from build123d import *

# Parameters (mm, degrees)
SKETCH1_R     = 4.7625
SKETCH1_R_2   = 4.0513
SHAFT_DEPTH   = 304.8
CUTAWAY_DEPTH = 305.874404981


with BuildPart() as part:
    # Sketch1 → Shaft (new body)
    with BuildSketch(Plane(origin=(0, 0, 0), x_dir=(1, 0, 0), z_dir=(0, 1, 0))):
        with Locations(Location((0, 0, 0), (0, 0, 270))):
            Circle(SKETCH1_R)
        with Locations(Location((0, 0, 0), (0, 0, 270))):
            Circle(SKETCH1_R_2, mode=Mode.SUBTRACT)
    extrude(amount=-SHAFT_DEPTH)

    # Sketch2 → Cutaway (cut, through all)
    with BuildSketch(Plane.XY):
        with BuildLine():
            Line((-1.27, -6.35), (1.27, -6.35))
            ThreePointArc((1.27, -6.35), (1.719012806, -6.164012806), (1.905, -5.715))
            Line((1.905, -5.715), (1.905, 0))
            Line((1.905, 0), (-1.905, 0))
            Line((-1.905, 0), (-1.905, -5.715))
            ThreePointArc((-1.905, -5.715), (-1.719012806, -6.164012806), (-1.27, -6.35))
        make_face()
    extrude(amount=-CUTAWAY_DEPTH, mode=Mode.SUBTRACT)


solid = part.part
Can you work these out from the model? Positions are in its coordinate system, mm. Give positions to 0.01 mm unless a question says otherwise; leave off trailing zeros. Order: outer loops, then holes, each group sorted by start corner. A loop starts at its lowest first (then second) coordinate and runs counter-clockwise, first axis right, second up. Notation, with made-up numbers: M 33,80.5 L 64,80.5 A24 ccw 64,114.5 Z; hole C 50.5,-8 d8. An arc over 180 degrees is marked long. Use one line per item in the form item = value. Start each with the question number.
Item 1: If we section it at B-B (y = -69.5): Write out the boundary of the cut face in (x, z) (1 decimal), then the cut area to 3 significant figures.
Item 2: We'd pull the mould along Z, two halves only. Please class faces 1 (the cylindrical face through (-2.9, -150.27, -3.78)), 2 (the flat face through (2, 0, 4)), 3 (the cylindrical face through (0.178, -150.266, -4.047)): +Z half, -Z half, draft (parallel to the pull), parting line (faces both ways), or undercut.
Item 3: If I drill on line 1 along X through (y, z) = (-242, 0); line 2 along X through (y, z) = (-190.5, 0.5); line 3 along Z through (x, y) = (3.5, -71.5), over which ranges is the centre line in solid material (lowest first)?
Item 4: If we section it at A-A (z = 0): Write out the boundary of the cut face in (x, y), then the cut area to 3 significant figures.
Item 5: Will these pins go through, and if not, where does the flat tip stop? pin 1 Ø1 at (x, z) = (0.5, 2.5) entering from -Y; pin 2 Ø2 at (y, z) = (-89, -3) entering from -X; pin 3 Ø0.7 at (x, z) = (-0.5, -4) entering from +Y; pin 4 Ø1.5 at (x, y) = (-2, -137.5) entering from -Z.
Outcome:
q1.outline = C 0,0 d9.5; hole C 0,0 d8.1
q1.area = 19.7 mm2
q2.face_1 = parting line
q2.face_2 = draft
q2.face_3 = undercut
q3.line_1 = -4.76 to -4.05, 4.05 to 4.76
q3.line_2 = -4.74 to -4.02, 4.02 to 4.74
q3.line_3 = -3.23 to -2.04, 2.04 to 3.23
q4.outline = M -4.76,-304.8 L -4.05,-304.8 L -4.05,0 L -4.76,0 Z; M 4.05,-304.8 L 4.76,-304.8 L 4.76,0 L 4.05,0 Z
q4.area = 434 mm2
q5.pin_1 = through
q5.pin_2 = -4.32
q5.pin_3 = -6.35
q5.pin_4 = -4.6
